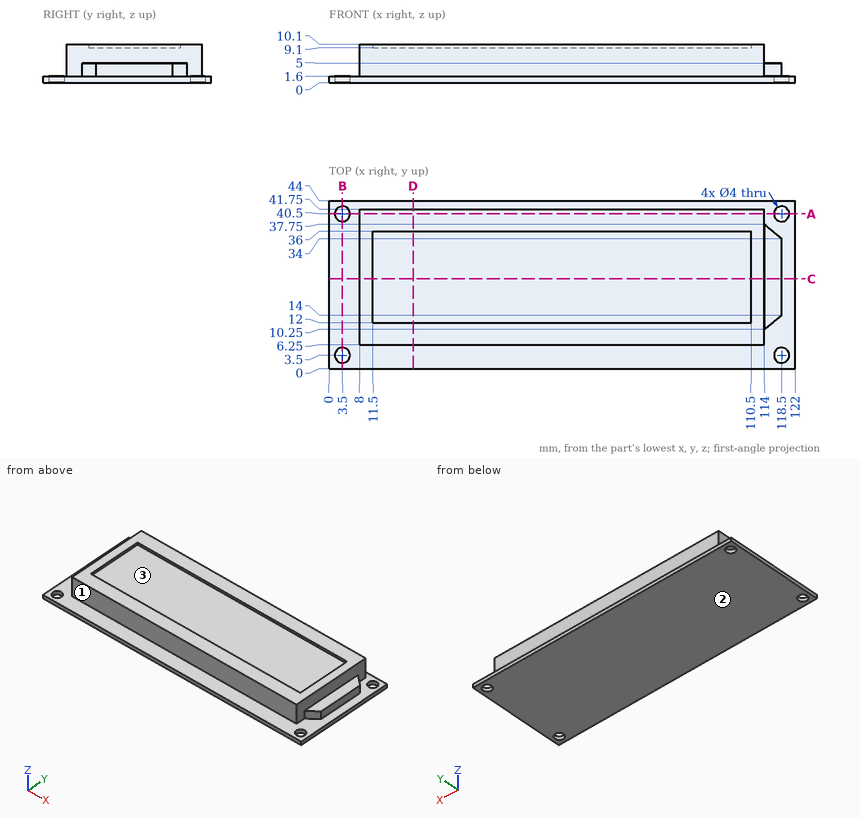
Job drawing, mm, ordinate dimensions from the low corner. One solid piece. Round coordinates to 2 decimals unless told otherwise and drop trailing zeros. Loops run counter-clockwise (first coordinate to the right, second up) from the corner with the lowest first, then second, coordinate; pieces in that order, holes last.
(1) Cut at B-B (x = 3.5). Give the cut face in (y, z), plus the area to 3 significant figures.
(2) Cut at D-D (x = 22). Give the cut face in (y, z).
(3) Cut at C-C (y = 23.5). Give the cut face in (x, z).
(4) Drop flat-ended pins along their axis: pin 1 (5 mm diameter, centred on x = 62.5, y = 24.5, fed in from +Z); pin 2 (0.5 mm diameter, centred on y = 26.5, z = 10, fed in from +X); pin 3 (5 mm diameter, centred on y = 17, z = 7, fed in from -X); pin 4 (3.5 mm diameter, centred on x = 118.5, y = 3.5, fed in from +Z). Give the stop position or say it passes through.
(5) Wall check: line 1 along Y through (x, z) = (118.5, 0.35); line 2 along Y through (x, z) = (57.5, 1.75); line 3 along Z through (x, y) = (89, 19). Give the ranges that are in metal, low to high.
(6) Cut at A-A (y = 40.5). Give the cut face in (x, z).
(7) Two-plate mould, pull along Y, no slides. Class the marked faces 1, 2 and 3: +Y half, -Y half, draft (parallel to the pull), parting line (faces both ways), or undercut.
Findings below:
1. outline: (0, 0) - (1.5, 0) - (1.5, 1.6) - (0, 1.6) - close; (5.5, 0) - (38.5, 0) - (38.5, 1.6) - (5.5, 1.6) - close; (42.5, 0) - (44, 0) - (44, 1.6) - (42.5, 1.6) - close
1. area: 57.6 mm2
2. outline: (0, 0) - (44, 0) - (44, 1.6) - (41.75, 1.6) - (41.75, 10.1) - (36, 10.1) - (36, 9.1) - (12, 9.1) - (12, 10.1) - (6.25, 10.1) - (6.25, 1.6) - (0, 1.6) - close
3. outline: (0, 0) - (122, 0) - (122, 1.6) - (118.5, 1.6) - (118.5, 5) - (114, 5) - (114, 10.1) - (110.5, 10.1) - (110.5, 9.1) - (11.5, 9.1) - (11.5, 10.1) - (8, 10.1) - (8, 1.6) - (0, 1.6) - close
4. pin 1: stops at z = 9.1
4. pin 2: stops at x = 114
4. pin 3: stops at x = 8
4. pin 4: passes through
5. line 1: y = 0 to 1.5, 5.5 to 38.5, 42.5 to 44
5. line 2: y = 6.25 to 41.75
5. line 3: z = 0 to 9.1
6. outline: (0, 0) - (1.5, 0) - (1.5, 1.6) - (0, 1.6) - close; (5.5, 0) - (116.5, 0) - (116.5, 1.6) - (114, 1.6) - (114, 10.1) - (8, 10.1) - (8, 1.6) - (5.5, 1.6) - close; (120.5, 0) - (122, 0) - (122, 1.6) - (120.5, 1.6) - close
7. face 1: -Y half
7. face 2: draft
7. face 3: undercut
